Verification items for this drawing (mm, ordinates from the low corner). A direction names the side the tool comes from. Round coordinates to 2 decimals unless told otherwise and drop trailing zeros. Loops run counter-clockwise (first coordinate to the right, second up) from the corner with the lowest first, then second, coordinate; pieces in that order, holes last. Notation, with made-up numbers: M 43.5,46.25 L 59.5,46.25 A5 cw 59.5,50.25 Z; hole C 69.25,18 d11. An arc over 180 degrees is marked long. Write item = value, one per line. Start each with the question number.
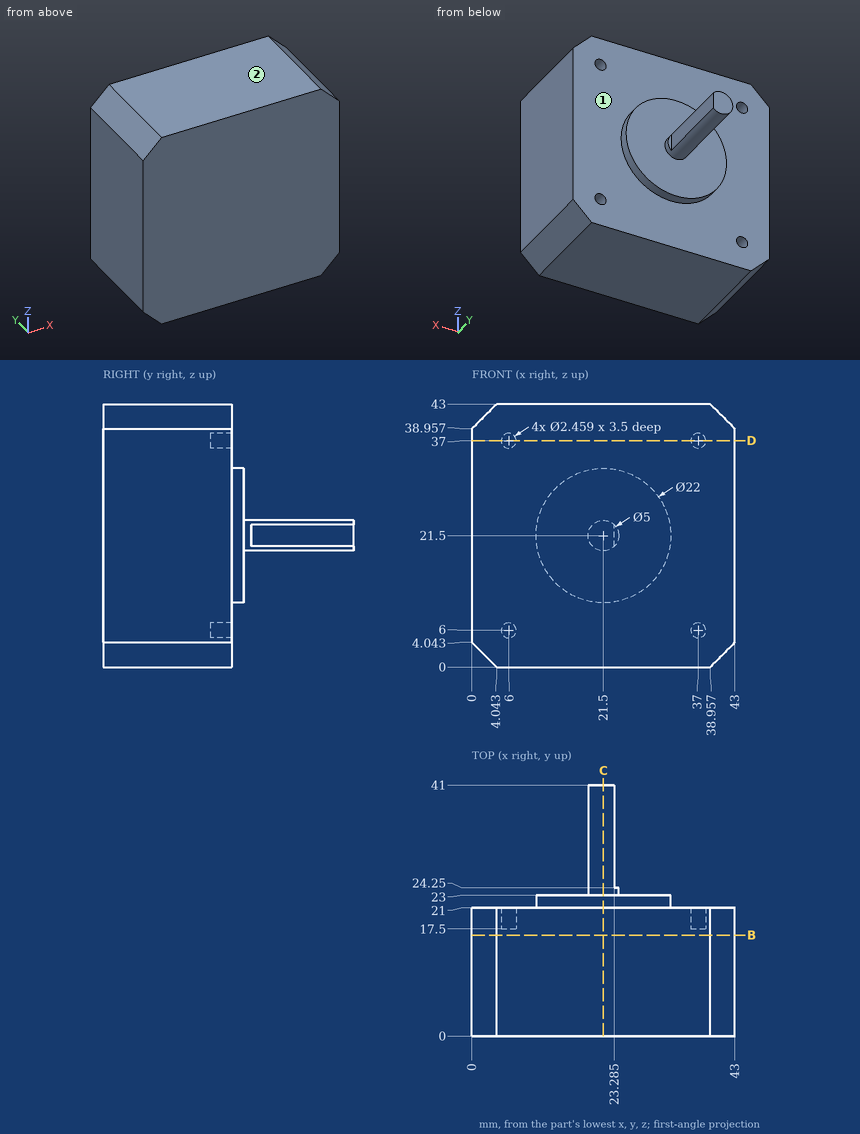
1. Section check C-C, the plane x = 21.5. Enter the section's corners in (y, z).
2. Thickness scan on line 1 (X direction, y = 19.55, z = 37); line 2 (Y direction, x = 21.5, z = 11). Record the ranges inside material, lowest first.
3. Gauge pin test, flat ends, axial feed: P1, Ø1.5, axis at y = 21, z = 25, coming from the -X side; P2, Ø1, axis at y = 27.5, z = 19.5, coming from the -X side; P3, Ø0.7, axis at x = 37, z = 37, coming from the +Y side; P4, Ø6, axis at x = 20.5, y = 34, coming from the +Z side. Record the tip position at first contact, or that the pin passes through.
4. Tool access check on the marked faces 1 and 2. Record the directions out of +Z, -Z, +X, -X, +Y, -Y that give a thin tool (end or side, any length) a straight path to the whole face; none if there is none.
5. Section check D-D, the plane z = 37. Enter the section's corners in (x, y).
6. Section check B-B, the plane y = 16.5. Enter the section's corners in (x, z), and give its area (3 significant figures).
Computed values:
q1.outline = M 0,0 L 21,0 L 21,10.5 L 23,10.5 L 23,19 L 41,19 L 41,24 L 23,24 L 23,32.5 L 21,32.5 L 21,43 L 0,43 Z
q2.line_1 = 0 to 4.77, 7.23 to 35.77, 38.23 to 43
q2.line_2 = 0 to 23
q3.P1 = 0
q3.P2 = 19.5
q3.P3 = 17.5
q3.P4 = 24
q4.face_1 = +Y
q4.face_2 = +Z, +X, -X, +Y, -Y
q5.outline = M 0,0 L 43,0 L 43,21 L 38.23,21 L 38.23,17.5 L 35.77,17.5 L 35.77,21 L 7.23,21 L 7.23,17.5 L 4.77,17.5 L 4.77,21 L 0,21 Z
q6.outline = M 0,4.04 L 4.04,0 L 38.96,0 L 43,4.04 L 43,38.96 L 38.96,43 L 4.04,43 L 0,38.96 Z
q6.area = 1,820 mm2
